Could you check a few things on this model? Use its own coordinates, in mm. Face numbers are marked on the shaded views. A direction names the side the tool comes from. Give positions to 0.01 mm unless a question says otherwise; leave off trailing zeros. Order: outer loops, then holes, each group sorted by start corner. A loop starts at its lowest first (then second) coordinate and runs counter-clockwise, first axis right, second up. Notation, with made-up numbers: M -5,87 L 9,87 A18 ccw 9,104 Z; hole C 35,-25 d4. An arc over 180 degrees is marked long. Use a Markdown table: item, result. Add a question column.
Item 1: Suppose I cut it at B-B on y = 66. Write out the boundary of the cut face in (x, z), plus the area to 3 significant figures.
Item 2: For the marked faces 5 and 6, which set-ups out of +Z, -Z, +X, -X, +Y, -Y let a thin tool reach every point of the face, with its end or its side?
Item 3: Suppose I cut it at A-A on z = -66.5. Write out the boundary of the cut face in (x, y).
Item 4: I'm going to push a flat-ended pin straight in: pin 1 Ø3 at (x, z) = (143, -71) entering from -Y. Where does the tip first touch, or does it pass through?
Item 5: If I drill on L1, parallel to X at y = 235.5, z = -78; L2, parallel to Z at x = 105.5, y = 271; L3, parallel to Y at x = 41.5, z = -24, over which ranges is the centre line in solid material (lowest first)? Write a range as from..to.
Item 6: Suppose I cut it at C-C on x = 39. Write out the boundary of the cut face in (y, z), plus the area to 3 significant figures.
Item 7: If we mould it in two halves opening along Z, with no side actions, what happens to the marked faces 1, 2, 3 and 4? For each: released by +Z, released by -Z, zero draft, split by the parting line, or undercut.
from build123d import *

# Parameters (mm, degrees)
SKETCH1_W           = 323.088
SKETCH1_H           = 89.916
BOSS_EXTRUDE1_DEPTH = 290.068
CUT_EXTRUDE1_START  = -5.08
SKETCH2_W           = 312.928
SKETCH2_H           = 79.756
CUT_EXTRUDE1_DEPTH  = 285.988


with BuildPart() as part:
    # Sketch1 → Boss-Extrude1 (new body)
    with BuildSketch(Plane(origin=(0, 0, 0), x_dir=(1, 0, 0), z_dir=(0, 1, 0))):
        with Locations((161.544, 44.958)):
            Rectangle(SKETCH1_W, SKETCH1_H)
    extrude(amount=BOSS_EXTRUDE1_DEPTH)

    # Sketch2 → Cut-Extrude1 (cut, through all)
    with BuildSketch(Plane(origin=(0, 290.068, 0), x_dir=(1, 0, 0), z_dir=(0, 1, 0)).offset(CUT_EXTRUDE1_START)):
        with Locations((161.544, 44.958)):
            Rectangle(SKETCH2_W, SKETCH2_H)
    extrude(amount=-CUT_EXTRUDE1_DEPTH, mode=Mode.SUBTRACT)


solid = part.part
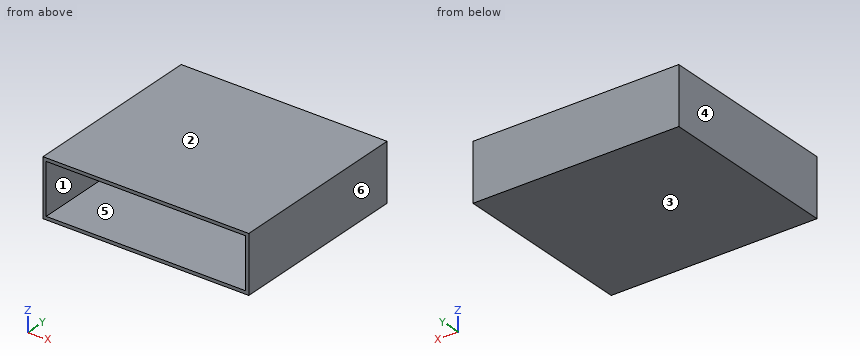
Findings below:
| question | item | result |
|---|---|---|
| 1 | outline | M 0,-89.92 L 323.09,-89.92 L 323.09,0 L 0,0 Z; hole M 5.08,-84.84 L 318.01,-84.84 L 318.01,-5.08 L 5.08,-5.08 Z |
| 1 | area | 4,090 mm^2 |
| 2 | face 5 | -Y |
| 2 | face 6 | +Z, -Z, +X, +Y, -Y |
| 3 | outline | M 0,0 L 5.08,0 L 5.08,284.99 L 318.01,284.99 L 318.01,0 L 323.09,0 L 323.09,290.07 L 0,290.07 Z |
| 4 | pin 1 | stops at y = 284.99 |
| 5 | L1 | x = 0..5.08, 318.01..323.09 |
| 5 | L2 | z = -89.92..-84.84, -5.08..0 |
| 5 | L3 | y = 284.99..290.07 |
| 6 | outline | M 0,-89.92 L 290.07,-89.92 L 290.07,0 L 0,0 L 0,-5.08 L 284.99,-5.08 L 284.99,-84.84 L 0,-84.84 Z |
| 6 | area | 3,350 mm^2 |
| 7 | face 1 | undercut |
| 7 | face 2 | released by +Z |
| 7 | face 3 | released by -Z |
| 7 | face 4 | zero draft |
